Design review of the part built by this model. Coordinates are the model's own, in mm. Face numbers are marked on the shaded views. A direction names the side the tool comes from. Give positions to 0.01 mm unless a question says otherwise; leave off trailing zeros. Order: outer loops, then holes, each group sorted by start corner. A loop starts at its lowest first (then second) coordinate and runs counter-clockwise, first axis right, second up.
Autodesk Inventor part; units mm, degrees
ref_plane "Work Plane2" through (3.35, 0, 0) normal (0, 0, -1) x (1, 0, 0)
ref_plane "YZ Plane" through (0, 0, 0) normal (1, 0, 0) x (0, 1, 0)
ref_plane "XZ Plane" through (0, 0, 0) normal (0, 1, 0) x (-1, 0, 0)
sketch "Sketch1" plane through (0, 0, 0) normal (0, 0, 1) x (1, 0, 0)
  line L0 (1.4, 0) -> (10, 0)
  line L1 (10, 0) -> (10, 1.5)
  line L2 (10, 1.5) -> (2.4, 1.5)
  line L3 (2.4, 1.5) -> (2.0933, 1.4)
  line L4 (2.0933, 1.4) -> (1.4, 1.4)
  line L5 (0, 2.75) -> (0, 1.3)
  line L6 (0, 1.3) -> (0.9645, 0.8191)
  line L7 (0.9645, 0.8191) -> (1.4, 0)
  line L8 (-2, 0) -> (12, 0)
  line L9 (0, -0.55) -> (0, 3.3)
  line L10 (0, 2.75) -> (0.05, 2.75)
  line L11 (0.05, 2.75) -> (1.4, 1.4)
  line L12 (2.4, 1.5) -> (1.3, 1.5) construction
  dimension "d1" = 7.6
  dimension "d2" = 3
  dimension "d3" = 2.8
  dimension "d4" = 2.6
  dimension "d5" = 26.5
  dimension "d6" = 62
  dimension "d7" = 1.4
  dimension "d8" = 0.3067
  dimension "d12" = 5.5
  dimension "d13" = 45
  dimension "d15" = 10
  dimension "d24" = 1.4
revolve "Body" add sketch "Sketch1" angle 360 about axis through (1.4, 0, 0) along (1, 0, 0) contours L7 L6 L5 L10 L11 L4 L3 L2 L1 L0
sketch "Sketch2" plane through (0, 0, 0) normal (-1, 0, 0) x (0, 0, 1)
  line L0 (0, 1.3) -> (0, 0) construction
  line L1 (0, 0) -> (1.3, 0) construction
  arc A0 (0.39, 0) -> (0, 0.39) centre (0, 0) ccw construction
  arc A1 (0.455, 0) -> (0, 0.455) centre (0, 0) ccw construction
  arc A2 (1.2462, 0.37) -> (0.37, 1.2462) centre (0, 0) ccw
  line L2 (0, 0) -> (0.9192, 0.9192) construction
  line L3 (0.37, 1.2462) -> (0.2393, 0.387)
  line L4 (1.2462, 0.37) -> (0.387, 0.2393)
  arc A3 (0.37, 1.2462) -> (0, 1.3) centre (0, 0) ccw
  arc A4 (1.3, 0) -> (1.2462, 0.37) centre (0, 0) ccw
  line L5 (0, -3.85) -> (0, 3.85)
  line L6 (-3.85, 0) -> (3.85, 0)
  arc A5 (0.37, -1.2462) -> (1.2462, -0.37) centre (0, 0) ccw
  line L7 (0.37, -1.2462) -> (0.2393, -0.387)
  line L8 (1.2462, -0.37) -> (0.387, -0.2393)
  arc A6 (0, -1.3) -> (0.37, -1.2462) centre (0, 0) ccw
  arc A7 (1.2462, -0.37) -> (1.3, 0) centre (0, 0) ccw
  arc A8 (-0.37, 1.2462) -> (-1.2462, 0.37) centre (0, 0) ccw
  line L9 (-0.37, 1.2462) -> (-0.2393, 0.387)
  line L10 (-1.2462, 0.37) -> (-0.387, 0.2393)
  arc A9 (0, 1.3) -> (-0.37, 1.2462) centre (0, 0) ccw
  arc A10 (-1.2462, 0.37) -> (-1.3, 0) centre (0, 0) ccw
  arc A11 (-0.37, -1.2462) -> (0, -1.3) centre (0, 0) ccw
  arc A12 (-1.2462, -0.37) -> (-0.37, -1.2462) centre (0, 0) ccw
  arc A13 (-1.3, 0) -> (-1.2462, -0.37) centre (0, 0) ccw
  line L11 (-1.2462, -0.37) -> (-0.387, -0.2393)
  line L12 (-0.37, -1.2462) -> (-0.2393, -0.387)
  arc A14 (0.2393, 0.387) -> (0.387, 0.2393) centre (0.3675, 0.3675) ccw
  arc A15 (0.387, -0.2393) -> (0.2393, -0.387) centre (0.3675, -0.3675) ccw
  arc A16 (-0.387, 0.2393) -> (-0.2393, 0.387) centre (-0.3675, 0.3675) ccw
  arc A17 (-0.2393, -0.387) -> (-0.387, -0.2393) centre (-0.3675, -0.3675) ccw
  point P0 (0.9192, -0.9192)
  point P1 (-0.9192, 0.9192)
  point P2 (-0.9192, -0.9192)
  dimension "d17" = 0.78
  dimension "d18" = 0.91
  dimension "d19" = 2.6
  dimension "d20" = 45
  dimension "d21" = 0.37
extrude "Slot" add sketch "Sketch2" against normal up to surface draft 5 contours L4 A14 L3 A2 | A5 L7 A15 L8 | L9 A16 L10 A8 | A12 L11 A17 L12
fillet "Fillet1" radius 0.148 4 edges at (0, 1.3, 0) (0, 0, -1.3) (0, -1.3, 0) (0, 0, 1.3)
thread "Thread"
ref_plane "Work Plane2" through (3.35, 0, 0) normal (0, 0, -1) x (1, 0, 0)
fillet "Fillet2" radius 0.2 1 edges at (1.4, -1.4, 0)
chamfer "Chamfer1" distance 0.3067 distance2 0.3067 1 edges at (10, -1.5, 0) measured on face at (10, -0.5112, 0.3316)
equation "\"d1\" = GEL"
equation "\"d2\" = GD"
equation "\"d3\" = BDM"
equation "\"d4\" = SDM"
equation "\"d7\" = INTI"
equation "\"d8\" = GAL"
equation "\"d12\" = KOD"
equation "\"d13\" = 0.5 * SEWI"
equation "\"d15\" = NLG"
equation "\"d24\" = KOH"
equation "\"d17\" = 0.3 * SDM"
equation "\"d18\" = 0.35 * SDM"
equation "\"d19\" = SDM"
equation "\"d21\" = 0.5 * SBR"
equation "\"d23\" = 0.2 * SBR"
equation "\"d10\" = GEL"
equation "\"d93\" = r"
equation "\"d94\" = -0.5 * SPD + 0.5 * GD"
equation "\"NLG\" = 10"
equation "\"GEL\" = -KOH + NLG - INA"
equation "\"GAL\" = 0.61345 * PTC"
equation "\"SPD\" = NND - 1.2269 * PTC"
equation "\"KOD\" = 5.5"
equation "\"KOH\" = 1.4"
equation "\"SBR\" = 0.74"
equation "\"INTI\" = 1.4"
equation "\"SDM\" = 2.6"
equation "\"GD\" = NND"
equation "\"BDM\" = 2.8"
equation "\"SEWI\" = 90deg"
equation "\"d9\" = SDM"
equation "\"GUL\" = 0.61345 * PTC"
equation "\"TOA\" = 30deg"
equation "\"PTC\" = 0.5"
equation "\"EPV\" = 1.8"
equation "\"THREADDIA\" = 3"
equation "\"FAWI\" = 90deg"
equation "\"RR\" = 0.4"
equation "\"KOHMIN\" = 1.26"
equation "\"NND\" = 3"
equation "\"GD1\" = THREADDIA - 1.2269 * PTC"
equation "\"INA\" = 1"
equation "\"r\" = 0.2"
properties part number "Screw GB/T 13806.1-1992 B M3 x 10" material "Steel, Mild-1"
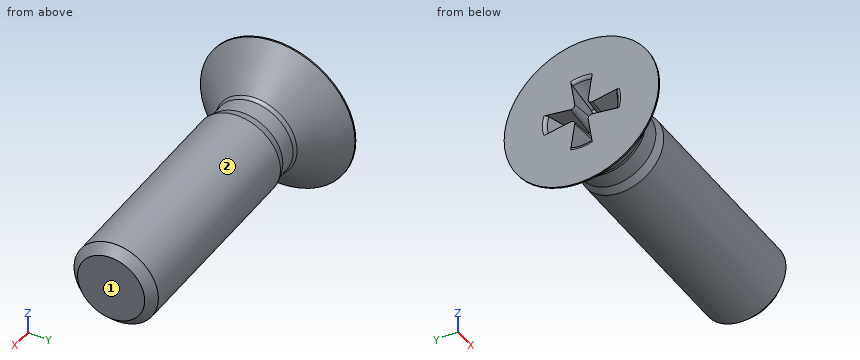
1. For line 1 along Y through (x, z) = (8.5, -0.35); line 2 along Y through (x, z) = (2, 0.15); line 3 along X through (y, z) = (1.35, 0.85), list the stretches that pass through material, from the lowest coordinate up.
Recorded:
line 1: y = -1.46 to 1.46
line 2: y = -1.39 to 1.39
line 3: x = 0 to 1.2
2. Machinability: for the marked faces 1 and 2, which of the approach directions +Z, -Z, +X, -X, +Y, -Y give a long, thin tool a straight path to every point of the face, cutting with its end or side? Answer none if there is none.
Recorded:
face 1: +Z, -Z, +X, +Y, -Y
face 2: +X
3. Take a section at B-B (x = 8.5). State the section outline as (y, z) points, then the cut area to 3 significant figures.
Recorded:
outline: circle Ø3 at (0, 0)
area: 7.07 mm2
4. For pin 1 (2 mm diameter, centred on x = 3, z = 0.5, fed in from +Y); pin 2 (2 mm diameter, centred on x = 4.5, z = 1.5, fed in from +Y), all flat-tipped, find the tip position at first contact; note any pin that passes through.
Recorded:
pin 1: stops at y = 1.5
pin 2: stops at y = 1.41
5. Take a section at A-A (x = 0.5). State the section outline as (y, z) points, then the cut area to 3 significant figures.
Recorded:
outline: circle Ø4.6 at (0, 0); hole (-1.01, -0.29) - (-0.39, -0.2) arc R0.17 cw to (-0.2, -0.39) - (-0.29, -1.01) arc R1.05 ccw to (0.29, -1.01) - (0.2, -0.39) arc R0.17 cw to (0.39, -0.2) - (1.01, -0.29) arc R1.05 ccw to (1.01, 0.29) - (0.39, 0.2) arc R0.17 cw to (0.2, 0.39) - (0.29, 1.01) arc R1.05 ccw to (-0.29, 1.01) - (-0.2, 0.39) arc R0.17 cw to (-0.39, 0.2) - (-1.01, 0.29) arc R1.05 ccw to start
area: 14.9 mm2
